```python
from build123d import *

# Parameters (mm, degrees)
SKETCH_4_R               = 13.5
EXTRUDE_1_DEPTH          = 1
CHAMFER_1_SIZE           = 2
CUT_EXTRUDE_1_DEPTH      = 65.031242374
PATTERN_CIRCULAR_1_COUNT = 6


with BuildPart() as part:
    # 草圖3 → 旋轉1 (revolve)
    with BuildSketch(Plane(origin=(0, 0, 0), x_dir=(0, 0, -1), z_dir=(1, 0, 0))):
        Polygon((0, 0), (15, 0), (15, 20), (26, 20), (26, 0), (40, 0), (40, -10), (0, -10), align=None)
    revolve(axis=Axis((0, -10, -40), (0, 0, 1)))

    # 草圖4 → 填料-伸長1 (add)
    with BuildSketch(Plane(origin=(0, 0, -26), x_dir=(-1, 0, 0), z_dir=(0, 0, -1))):
        with Locations(Location((0, -10, 0), (0, 0, 90))):
            Circle(SKETCH_4_R)
    extrude(amount=EXTRUDE_1_DEPTH)

    # 導角1
    chamfer_1_edges = [part.edges().sort_by_distance(p)[0] for p in [
        (0, -20, -40),
        (0, -20, 0),
    ]]
    chamfer(chamfer_1_edges, length=CHAMFER_1_SIZE)

    # 草圖1 → 除料-伸長1 (cut, through all)
    with BuildSketch(Plane.XY):
        with BuildLine():
            Line((-3.988148122, 15.692307692), (-3.988148122, 19.733729577))
            ThreePointArc((-3.988148122, 19.733729577), (13.235915698, 16.922305541), (25.980762114, 5))
            ThreePointArc((25.980762114, 5), (13.7123081, 11.179459253), (0, 12))
            ThreePointArc((0, 12), (-2.717464882, 13.064802457), (-3.988148122, 15.692307692))
        make_face()
    cut_extrude_1 = extrude(amount=-CUT_EXTRUDE_1_DEPTH, mode=Mode.SUBTRACT)

    # 環狀複製排列1: 除料-伸長1 ×6 about axis
    pattern_circular_1_axis = Axis((0, -10, 0), (0, 0, 1))
    for i in range(1, PATTERN_CIRCULAR_1_COUNT):
        add(cut_extrude_1.rotate(pattern_circular_1_axis, i * 360 / PATTERN_CIRCULAR_1_COUNT), mode=Mode.SUBTRACT)


solid = part.part
```
For this review, take the finished solid that the model builds, in its own axes (mm). A direction names the side the tool comes from. Coordinates: 2 decimals unless noted, no trailing zeros. Write each loop counter-clockwise with the first axis right and the second up, starting at its lowest first coordinate (ties: lowest second). Pieces come first, ordered by that corner, then holes.
(1) Wall thickness on probe 1 along Z at (x, y) = (-4, 11.5); probe 2 along X at (y, z) = (-10, -9.5); probe 3 along Y at (x, z) = (-0.5, -4): over which ranges is each line inside the solid? List them lowest first.
(2) Add section D-D on z = -34. Give the boundary of the cut face in (x, y), then the cut area to 3 significant figures.
(3) Add section A-A on z = -17. Give the boundary of the cut face in (x, y), then the cut area to 3 significant figures.
(4) The part is to be moulded in two halves that separate along X. For faces 1 (the face through (18.607, 3.845, -20.423)), 2 (the face through (-25.3, 0, -20.4)), 3 (the face through (-3, -0.46, -32.58)), 4 (the face through (-12, -17, -26)), say which applies: +X half, -X half, draft (parallel to the pull), parting line (faces both ways), or undercut.
(5) Tool access review of faces 5 (the face through (-3, -0.46, -8.59)), 6 (the face through (-24.612, -10.674, -20.423)), 7 (the face through (-5.17, 2.47, -26.49)), 8 (the face through (2.69, -33.04, -20.42)): name each direction out of +Z, -Z, +X, -X, +Y, -Y from which nothing blocks a thin tool from reaching the whole face with its end or side.
(6) Add section B-B on x = 12.5. Give the boundary of the cut face in (y, z).
(7) For pin 1 Ø2.5 at (y, z) = (-37, -20.5) entering from -X; pin 2 Ø1 at (x, z) = (-11.5, -15.5) entering from -Y; pin 3 Ø2 at (x, y) = (1, -29.5) entering from -Z, all flat-tipped, find the tip position at first contact; note any pin that passes through.
(8) Add section C-C on y = -10. Give the boundary of the cut face in (x, z), then the cut area to 3 significant figures.
Answer sheet:
1. probe 1: z = -26 to -15
1. probe 2: x = -10 to 10
1. probe 3: y = -19.99 to -0.01
2. outline: circle Ø20 at (0, -10)
2. area: 314 mm2
3. outline: (-26.34, 0.6) arc R34 ccw to (-19.05, -21) arc R4 cw to (-20.26, -26.3) - (-22.35, -27.51) arc R34 ccw to (0, -32) arc R4 cw to (3.99, -35.69) - (3.99, -38.11) arc R34 ccw to (19.05, -21) arc R4 cw to (24.24, -19.39) - (26.34, -20.6) arc R34 ccw to (19.05, 1) arc R4 cw to (20.26, 6.3) - (22.35, 7.51) arc R34 ccw to (0, 12) arc R4 cw to (-3.99, 15.69) - (-3.99, 18.11) arc R34 ccw to (-19.05, 1) arc R4 cw to (-24.24, -0.61) - close
3. area: 1,870 mm2
4. face 1: +X half
4. face 2: undercut
4. face 3: parting line
4. face 4: draft
5. face 5: +Z
5. face 6: +Z, -Z, -X
5. face 7: -Z
5. face 8: +Z, -Z, -Y
6. outline: (-31.41, -26) - (-15.1, -26) - (-15.1, -27) - (-4.9, -27) - (-4.9, -26) - (11.48, -26) - (11.48, -15) - (-31.41, -15) - close
7. pin 1: stops at x = 3.99
7. pin 2: stops at y = -31.79
7. pin 3: stops at z = -26
8. outline: (-24.83, -26) - (-13.5, -26) - (-13.5, -27) - (-10, -27) - (-10, -38) - (-8, -40) - (8, -40) - (10, -38) - (10, -27) - (13.5, -27) - (13.5, -26) - (24.83, -26) - (24.83, -15) - (10, -15) - (10, -2) - (8, 0) - (-8, 0) - (-10, -2) - (-10, -15) - (-24.83, -15) - close
8. area: 1,130 mm2
